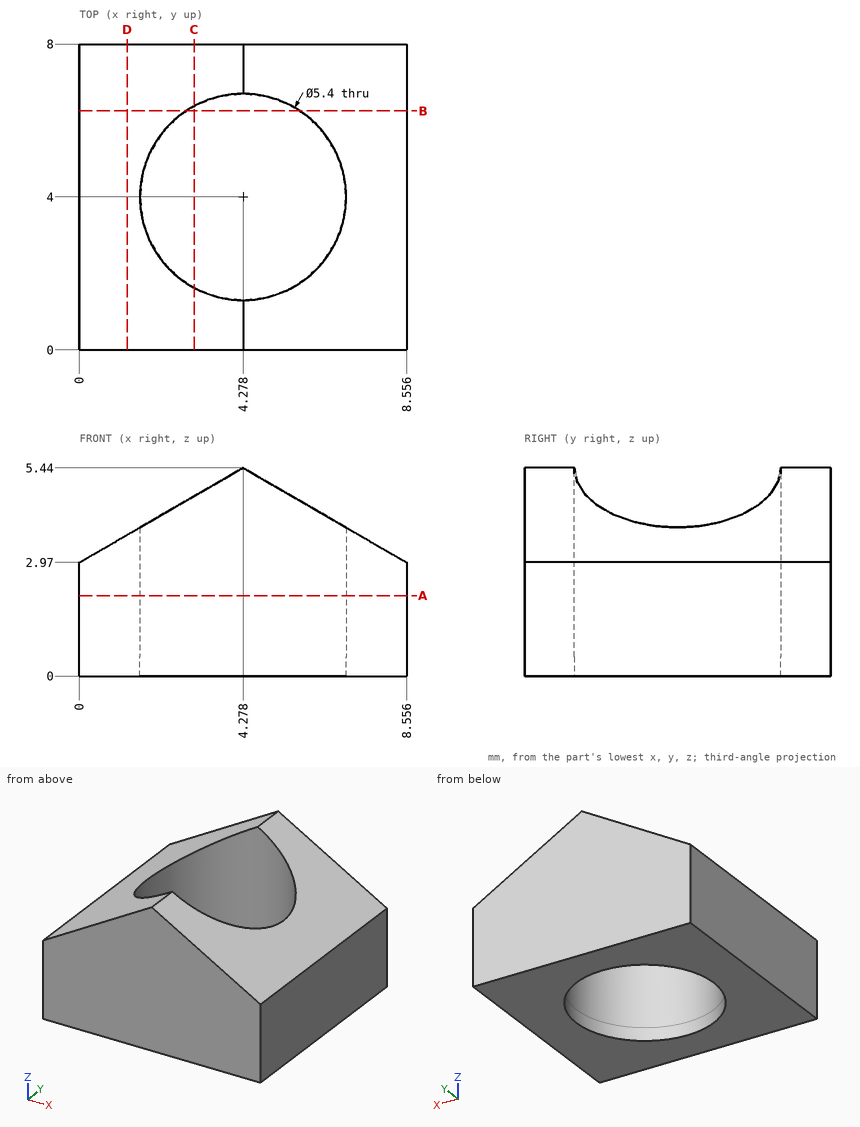
Print and shaded views of the part. All mm, measured from the part's lowest x, y and z. Coordinates: 2 decimals unless noted, no trailing zeros. Loops run counter-clockwise (first coordinate to the right, second up) from the corner with the lowest first, then second, coordinate; pieces in that order, holes last. Notation, with made-up numbers: (41, 4.25) -> (95, 4.25) arc R16 ccw to (95, 32.25) -> close; hole circle Ø4 at (70.25, 0.5). An arc over 180 degrees is marked (long way). Use a Markdown table: item, result. Add a question column.
Item 1: Band-saw the part on B-B on y = 6.25. Write the cut outline in (x, z).
Item 2: Probe probe 1 along X at (y, z) = (4, 0.25); probe 2 along Y at (x, z) = (4.25, 1.5); probe 3 along Y at (x, z) = (5.75, 3.1) (1 decimal). List the from-to ranges inside material, lowest first.
Item 3: Band-saw the part on C-C on x = 3. Write the cut outline in (y, z).
Item 4: Band-saw the part on D-D on x = 1.25. Write the cut outline in (y, z).
Item 5: Band-saw the part on A-A on z = 2.1. Write the cut outline in (x, y).
Item 6: Flat gauge pin, fed straight in: P1, Ø3, axis at x = 4.28, y = 4, coming from the -Z side. Where does the tip first touch, or does it go through?
Geometry says:
| question | item | result |
|---|---|---|
| 1 | outline | (0, 0) -> (2.79, 0) -> (2.79, 4.58) -> (0, 2.97) -> close; (5.77, 0) -> (8.56, 0) -> (8.56, 2.97) -> (5.77, 4.58) -> close |
| 2 | probe 1 | 0 to 1.58, 6.98 to 8.56 |
| 2 | probe 2 | 0 to 1.3, 6.7 to 8 |
| 2 | probe 3 | 0 to 1.7, 6.3 to 8 |
| 3 | outline | (0, 0) -> (1.62, 0) -> (1.62, 4.7) -> (0, 4.7) -> close; (6.38, 0) -> (8, 0) -> (8, 4.7) -> (6.38, 4.7) -> close |
| 4 | outline | (0, 0) -> (8, 0) -> (8, 3.69) -> (0, 3.69) -> close |
| 5 | outline | (0, 0) -> (8.56, 0) -> (8.56, 8) -> (0, 8) -> close; hole circle Ø5.4 at (4.28, 4) |
| 6 | P1 | through |
